Could you check a few things on this model? Use its own coordinates, in mm. A direction names the side the tool comes from. Coordinates: 2 decimals unless noted, no trailing zeros. Loops run counter-clockwise (first coordinate to the right, second up) from the corner with the lowest first, then second, coordinate; pieces in that order, holes last. Notation, with made-up numbers: (88, 86) - (147, 86) arc R22 cw to (147, 124) - close; hole circle Ø5 at (0.25, -10). An arc over 180 degrees is marked (long way). Put each result on its own line as item: value. Start each with the question number.
```python
from build123d import *

# Parameters (mm, degrees)
BOSS_EXTRUDE1_DEPTH     = 92
FILLET1_R               = 6
SKETCH2_R               = 2.05
CUT_EXTRUDE1_DEPTH      = 93.86549413
LPATTERN1_COUNT         = 5
LPATTERN1_PITCH         = 8
MIRROR1_COPY_1_SKETCH_R = 2.05
MIRROR1_COPY_1_DEPTH    = 93.86549413
MIRROR1_COPY_2_SKETCH_R = 2.05
MIRROR1_COPY_2_DEPTH    = 93.86549413
MIRROR1_COPY_3_SKETCH_R = 2.05
MIRROR1_COPY_3_DEPTH    = 93.86549413
MIRROR1_COPY_4_SKETCH_R = 2.05
MIRROR1_COPY_4_DEPTH    = 93.86549413


with BuildPart() as part:
    # Sketch1 → Boss-Extrude1 (new body)
    with BuildSketch(Plane.XY):
        Polygon((0, 0), (4, 0), (4, 2), (3, 2), (3, 10), (4, 10), (4, 12), (0, 12), align=None)
    extrude(amount=-BOSS_EXTRUDE1_DEPTH)

    # Fillet1
    fillet1_edges = [part.edges().sort_by_distance(p)[0] for p in [
        (2, 12, 0),
        (2, 0, 0),
        (2, 0, -92),
        (2, 12, -92),
    ]]
    fillet(fillet1_edges, radius=FILLET1_R - 0.0001)  # a hair under: the kernel refuses the full size

    # Sketch2 → Cut-Extrude1 (cut, through all)
    with BuildSketch(Plane.ZY):
        with Locations(Location((-86, 6, 0), (0, 0, 270))):
            Circle(SKETCH2_R)
    cut_extrude1 = extrude(amount=-CUT_EXTRUDE1_DEPTH, mode=Mode.SUBTRACT)

    # LPattern1: Cut-Extrude1 ×5
    with Locations(*[(0, 0, i * LPATTERN1_PITCH) for i in range(1, LPATTERN1_COUNT)]):
        add(cut_extrude1, mode=Mode.SUBTRACT)

    # Mirror1: Cut-Extrude1 across plane
    add(cut_extrude1.mirror(Plane.XY.offset(-46)), mode=Mode.SUBTRACT)

    # Mirror1 copy 1 sketch → Mirror1 copy 1 (cut, through all)
    with BuildSketch(Plane(origin=(0, 0, -100), x_dir=(0, 0, -1), z_dir=(-1, 0, 0))):
        with Locations((-86, -6)):
            Circle(MIRROR1_COPY_1_SKETCH_R)
    extrude(amount=-MIRROR1_COPY_1_DEPTH, mode=Mode.SUBTRACT)

    # Mirror1 copy 2 sketch → Mirror1 copy 2 (cut, through all)
    with BuildSketch(Plane(origin=(0, 0, -108), x_dir=(0, 0, -1), z_dir=(-1, 0, 0))):
        with Locations((-86, -6)):
            Circle(MIRROR1_COPY_2_SKETCH_R)
    extrude(amount=-MIRROR1_COPY_2_DEPTH, mode=Mode.SUBTRACT)

    # Mirror1 copy 3 sketch → Mirror1 copy 3 (cut, through all)
    with BuildSketch(Plane(origin=(0, 0, -116), x_dir=(0, 0, -1), z_dir=(-1, 0, 0))):
        with Locations((-86, -6)):
            Circle(MIRROR1_COPY_3_SKETCH_R)
    extrude(amount=-MIRROR1_COPY_3_DEPTH, mode=Mode.SUBTRACT)

    # Mirror1 copy 4 sketch → Mirror1 copy 4 (cut, through all)
    with BuildSketch(Plane(origin=(0, 0, -124), x_dir=(0, 0, -1), z_dir=(-1, 0, 0))):
        with Locations((-86, -6)):
            Circle(MIRROR1_COPY_4_SKETCH_R)
    extrude(amount=-MIRROR1_COPY_4_DEPTH, mode=Mode.SUBTRACT)


solid = part.part
```
(1) I need wall thicknesses on L1, parallel to Y at x = 3.35, z = -20; L2, parallel to Y at x = 1.75, z = -14; L3, parallel to X at y = 6, z = -25. Which ranges of each line are inside material? Lowest first, please. Write a range as [from, to].
(2) Which directions (+Z, -Z, +X, -X, +Y, -Y) give clear straight access to the entire face, cutting with the end or side of a thin tool? Please do faces 1 (the cylindrical face through (1.972, 10.289, -1.804)), 2 (the flat face through (3, 6, -45)).
(3) I want a section at A-A on z = -78. List the corners of the cut face in (x, y) for me.
(4) For pin 1 Ø5.5 at (y, z) = (6, -14) entering from +X, with a flat end and sliding along its axis, tell me the tip position at first contact or that it passes through.
(5) If we mould it in two halves opening along Z, with no side actions, what happens to faces 3 (the flat face through (4, 1, -45)), 4 (the cylindrical face through (1.972, 10.289, -90.196)), 5 (the cylindrical face through (1.479, 6.267, -67.967))? For each: pulls with the +Z half, pulls with the -Z half, needs draft (parallel to the pull), parting line crosses it, or undercut.
(6) I want a section at B-B on x = 2.15. Count the separate pieces of the cut face and the enclosed holes in it, and give its area (3 significant figures).
Answer sheet:
1. L1: y = [0, 2], [10, 12]
1. L2: y = [0, 3.95], [8.05, 12]
1. L3: x = [0, 3]
2. face 1: +Z, +X, -X, +Y
2. face 2: +Z, -Z, +X
3. outline: (0, 0) - (4, 0) - (4, 2) - (3, 2) - (3, 3.95) - (0, 3.95) - close; (0, 8.05) - (3, 8.05) - (3, 10) - (4, 10) - (4, 12) - (0, 12) - close
4. pin 1: stops at x = 3
5. face 3: needs draft
5. face 4: pulls with the -Z half
5. face 5: undercut
6. separate pieces: 1
6. enclosed holes: 10
6. area: 941 mm^2
